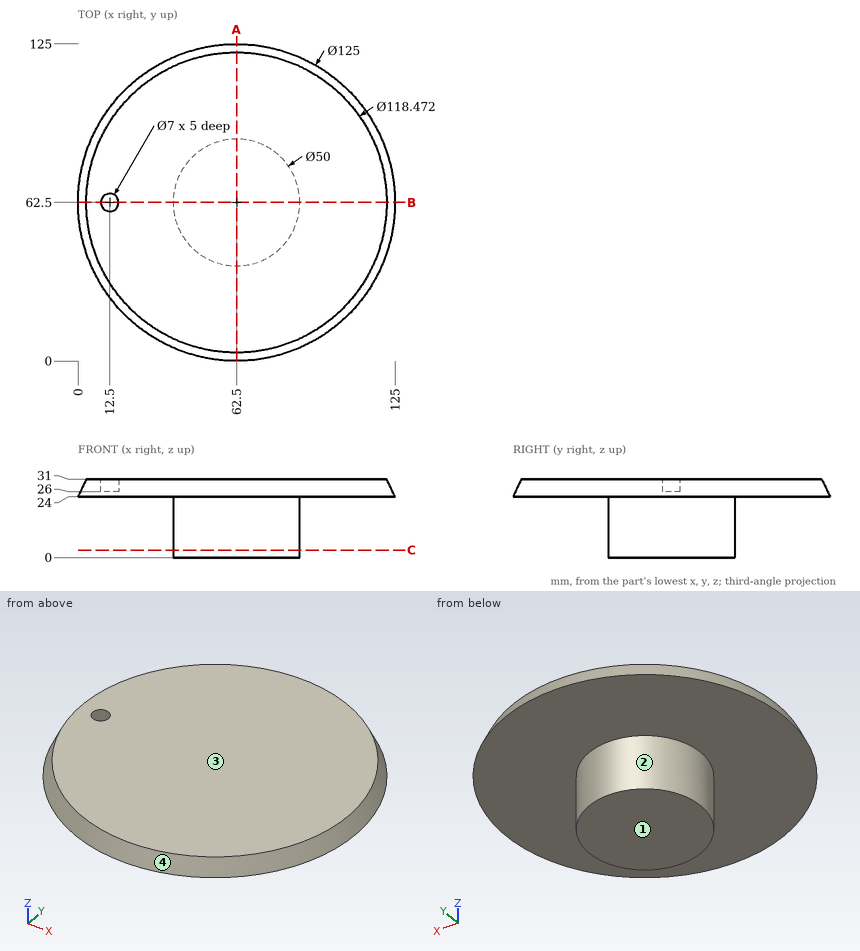
Answer from the drawing. Dimensions are ordinates in mm from the lowest x, y and z of the part. A direction names the side the tool comes from. Give positions to 0.01 mm unless a question says otherwise; leave off trailing zeros. Order: outer loops, then holes, each group sorted by start corner. A loop starts at its lowest first (then second) coordinate and runs counter-clockwise, first axis right, second up.
(1) Find section C-C (z = 3). Give the vertices of the cut face in (x, y), plus the area to 3 significant figures.
(2) Given pin 1 (12 mm diameter, centred on x = 41, z = 11.5, fed in from -Y) (1 decimal); pin 2 (8 mm diameter, centred on x = 12.5, y = 62.5, fed in from +Z); pin 3 (4 mm diameter, centred on x = 63, z = 18, fed in from +Y); pin 4 (2 mm diameter, centred on x = 54, z = 7.5, fed in from +Y), each flat-ended and moving along its own axis, determine where each tip first touches the part or whether it passes through.
(3) Find section A-A (x = 62.5). Give the vertices of the cut face in (y, z), plus the area to 3 significant figures.
(4) For the marked faces 1 and 2, determine the directions among +Z, -Z, +X, -X, +Y, -Y from which every point of the face is accessible in a straight line to the end or side of a thin tool.
(5) Straight lines are drawn through the part: L1, parallel to Y at x = 12.5, z = 28.8; L2, parallel to Z at x = 111, y = 33; L3, parallel to Y at x = 12.5, z = 27.1. For each, find the intervals that lie inside material, in ascending order.
(6) For a pull along Y with two mould halves and no side action, classify the marked faces 3 and 4 as released by +Y, released by -Y, zero draft, split by the parting line, or undercut.
(7) Find section B-B (y = 62.5). Give the vertices of the cut face in (x, z).
Result sheet:
1. outline: circle Ø50 at (62.5, 62.5)
1. area: 1,960 mm2
2. pin 1: stops at y = 42.9
2. pin 2: stops at z = 31
2. pin 3: stops at y = 87.5
2. pin 4: stops at y = 86.35
3. outline: (0, 24) - (37.5, 24) - (37.5, 0) - (87.5, 0) - (87.5, 24) - (125, 24) - (121.74, 31) - (3.26, 31) - close
3. area: 2,050 mm2
4. face 1: -Z, +X, -X, +Y, -Y
4. face 2: -Z
5. L1: y = 28.86 to 59, 66 to 96.14
5. L2: z = 24 to 31
5. L3: y = 27.46 to 59, 66 to 97.54
6. face 3: zero draft
6. face 4: split by the parting line
7. outline: (0, 24) - (37.5, 24) - (37.5, 0) - (87.5, 0) - (87.5, 24) - (125, 24) - (121.74, 31) - (16, 31) - (16, 26) - (9, 26) - (9, 31) - (3.26, 31) - close
